from build123d import *

# Parameters (mm, degrees)
SKETCH_R     = 5.5
PAD_DEPTH    = 3
SKETCH001_W  = 30
SKETCH001_H  = 20
PAD001_DEPTH = 5
SKETCH002_R  = 4.5
PAD002_DEPTH = 30
SKETCH003_W  = 20
SKETCH003_H  = 19
POCKET_DEPTH = 20.001
SKETCH004_W  = 4
SKETCH004_H  = 5
PAD003_DEPTH = 6


with BuildPart() as part:
    # Sketch → Pad (new body)
    with BuildSketch(Plane.XY):
        Circle(SKETCH_R)
    extrude(amount=PAD_DEPTH)

    # Sketch001 (on Face3 of Pad) → Pad001 (join)
    with BuildSketch(Plane.XY.offset(3)):
        with Locations((0, 4.5)):
            Rectangle(SKETCH001_W, SKETCH001_H)
    extrude(amount=PAD001_DEPTH)

    # Sketch002 (on Face6 of Pad001) → Pad002 (join)
    with BuildSketch(Plane.YZ.offset(15)):
        Polygon((-5.5, 7), (14.5, 7), (14.5, 8), (7.5, 27), (-2.5, 27), (-5.5, 8), align=None)
        with Locations((2.5, 20)):
            Circle(SKETCH002_R, mode=Mode.SUBTRACT)
    extrude(amount=-PAD002_DEPTH)

    # Sketch003 (on Face5 of Pad002) → Pocket (cut, through all)
    with BuildSketch(Plane.XZ.offset(5.5)):
        with Locations((0, 17.5)):
            Rectangle(SKETCH003_W, SKETCH003_H)
    extrude(amount=-POCKET_DEPTH, mode=Mode.SUBTRACT)

    # Sketch004 (on DatumPlane) → Pad003 (join)
    with BuildSketch(Plane(origin=(0, 0, 3), x_dir=(1, 0, 0), z_dir=(0, 0, -1))):
        Polygon((-15, 2), (-21, -1), (-21, -8), (-15, -11), (15, -11), (21, -8), (21, -1), (15, 2), align=None)
        with Locations((-17, -4.5)):
            Rectangle(SKETCH004_W, SKETCH004_H, mode=Mode.SUBTRACT)
        with Locations((17, -4.5)):
            Rectangle(SKETCH004_W, SKETCH004_H, mode=Mode.SUBTRACT)
    extrude(amount=-PAD003_DEPTH)


solid = part.part
Could you check a few things on this model? Use its own coordinates, in mm. A direction names the side the tool comes from. Give positions to 0.01 mm unless a question says otherwise; leave off trailing zeros. Order: outer loops, then holes, each group sorted by start corner. A loop starts at its lowest first (then second) coordinate and runs counter-clockwise, first axis right, second up. Notation, with made-up numbers: (-5.5, -2) -> (46.5, -2) arc R18 ccw to (46.5, 14) -> close; hole circle Ø10 at (-15, 39). An arc over 180 degrees is marked (long way). Return JSON: item names as keys, results as strings.
1. Imagine slicing it at D-D on z = 20. List the corners of the cut face in (x, y) for me, then the cut area to 3 significant figures.
Answer list:
{"outline": "(-15, -3.61) -> (-10, -3.61) -> (-10, -2) -> (-15, -2) -> close; (-15, 7) -> (-10, 7) -> (-10, 10.08) -> (-15, 10.08) -> close; (10, -3.61) -> (15, -3.61) -> (15, -2) -> (10, -2) -> close; (10, 7) -> (15, 7) -> (15, 10.08) -> (10, 10.08) -> close", "area": "46.8 mm2"}
2. Imagine slicing it at A-A on x = 12. List the corners of the cut face in (y, z) for me.
Answer list:
{"outline": "(-5.5, 3) -> (14.5, 3) -> (14.5, 8) -> (7.5, 27) -> (-2.5, 27) -> (-5.5, 8) -> close; hole circle Ø9 at (2.5, 20)"}
3. For pin 1 Ø4 at (x, y) = (2.5, 1.5) entering from +Z; pin 2 Ø9.5 at (y, z) = (4, 17) entering from -X; pin 3 Ø6 at (x, y) = (-14, 7) entering from -Z, each with a flat end and sliding along its axis, tell me the tip position at first contact or that it passes through.
Answer list:
{"pin 1": "stops at z = 9", "pin 2": "stops at x = -15", "pin 3": "stops at z = 3"}
4. Imagine slicing it at B-B on y = 0. List the corners of the cut face in (x, z) for me, then the cut area to 3 significant figures.
Answer list:
{"outline": "(-19, 3) -> (-5.5, 3) -> (-5.5, 0) -> (5.5, 0) -> (5.5, 3) -> (19, 3) -> (19, 9) -> (15, 9) -> (15, 16.26) -> (10, 16.26) -> (10, 9) -> (-10, 9) -> (-10, 16.26) -> (-15, 16.26) -> (-15, 9) -> (-19, 9) -> close; (-15, 23.74) -> (-10, 23.74) -> (-10, 27) -> (-15, 27) -> close; (10, 23.74) -> (15, 23.74) -> (15, 27) -> (10, 27) -> close", "area": "366 mm2"}
5. I need wall thicknesses on line 1 (X direction, y = -3, z = 22.25); line 2 (Z direction, x = -11, y = 2.5); line 3 (Z direction, x = -8, y = -3.5). Which ranges of each line are inside material? Lowest first, please. Write a range as from..to.
Answer list:
{"line 1": "x = -15..-10, 10..15", "line 2": "z = 3..15.5, 24.5..27", "line 3": "z = 3..8"}
6. Thinking about a two-plate mould opening in Y: for faces 1 (the flat face through (0.1, -2, 8.5)), 2 (the flat face through (-10, 4, 15)), 3 (the flat face through (-17, 2, 6)), which applies, pulls with the +Y half, pulls with the -Y half, needs draft (parallel to the pull), parting line crosses it, or undercut?
Answer list:
{"face 1": "pulls with the -Y half", "face 2": "needs draft", "face 3": "undercut"}
7. Imagine slicing it at C-C on x = -7. List the corners of the cut face in (y, z) for me.
Answer list:
{"outline": "(-5.5, 3) -> (14.5, 3) -> (14.5, 8) -> (11, 8) -> (11, 9) -> (-2, 9) -> (-2, 8) -> (-5.5, 8) -> close"}
8. On a 3-axis mill with a long thin cutter (end or side, diameter ignored), from which of +Z, -Z, +X, -X, +Y, -Y can I reach the whole of each face in a straight line? I mean faces 4 (the flat face through (-19.4, 4.4, 9)), 5 (the flat face through (0, -4, 8)), 6 (the flat face through (-0.1, 11, 8.5)), 7 (the flat face through (17, 2, 6)). Say none if no direction works.
Answer list:
{"face 4": "+Z, -X, +Y, -Y", "face 5": "+Z, -Y", "face 6": "+Z, +Y", "face 7": "+Z, -Z"}
